```python
from build123d import *

# Parameters (mm, degrees)
SKETCH1_W           = 39.1
SKETCH1_H           = 23
BOSS_EXTRUDE1_DEPTH = 5.5
CUT_EXTRUDE1_DEPTH  = 26.208183195
FILLET1_R           = 6.35
FILLET2_R           = 0.5
SKETCH3_W           = 9
SKETCH3_H           = 9
BOSS_EXTRUDE2_DEPTH = 6.35


with BuildPart() as part:
    # Sketch1 → Boss-Extrude1 (new, symmetric)
    with BuildSketch(Plane.XY):
        Rectangle(SKETCH1_W, SKETCH1_H)
    extrude(amount=BOSS_EXTRUDE1_DEPTH, both=True)

    # Sketch2 → Cut-Extrude1 (cut, through all)
    with BuildSketch(Plane.XY.offset(5.5)):
        Polygon((19.55, -11.5), (-2.05, -11.5), (-2.05, -0.389755132), (19.55, 1.5), align=None)
    extrude(amount=-CUT_EXTRUDE1_DEPTH, mode=Mode.SUBTRACT)

    # Fillet1
    fillet1_edges = [part.edges().sort_by_distance(p)[0] for p in [
        (-2.05, -0.389755132, 0),
    ]]
    fillet(fillet1_edges, radius=FILLET1_R)

    # Fillet2
    fillet2_edges = [part.edges().sort_by_distance(p)[0] for p in [
        (0, 11.5, 5.5),
        (19.55, 6.5, -5.5),
        (19.55, 6.5, 5.5),
        (19.55, 1.5, 0),
        (-2.05, -11.5, 0),
        (11.648280517, 0.808689123, -5.5),
        (11.648280517, 0.808689123, 5.5),
        (-2.05, -8.854229044, 5.5),
        (-2.05, -8.854229044, -5.5),
        (-0.381711089, -1.918460269, 5.5),
        (-0.381711089, -1.918460269, -5.5),
        (-19.55, 0, 5.5),
        (0, 11.5, -5.5),
        (-10.8, -11.5, -5.5),
        (-19.55, 0, -5.5),
        (-10.8, -11.5, 5.5),
        (-19.55, 11.5, 0),
        (19.55, 11.5, 0),
        (-19.55, -11.5, 0),
    ]]
    fillet(fillet2_edges, radius=FILLET2_R)

    # Sketch3 → Boss-Extrude2 (add)
    with BuildSketch(Plane(origin=(19.55, 0, 0), x_dir=(0, 0, -1), z_dir=(1, 0, 0))):
        with Locations((0, 6.479082794)):
            Rectangle(SKETCH3_W, SKETCH3_H)
    extrude(amount=BOSS_EXTRUDE2_DEPTH)


solid = part.part
```
Build history of the part. All positions in model axes, mm. A direction names the side the tool comes from. Coordinates: 2 decimals unless noted, no trailing zeros. Order: outer loops, then holes, each group sorted by start corner. A loop starts at its lowest first (then second) coordinate and runs counter-clockwise, first axis right, second up. Notation, with made-up numbers: M 56,-16 L 74,-16 A20 ccw 74,-4 Z; hole C -4,51 d6. An arc over 180 degrees is marked long. One line per question, with ' | ' between items. Start each with the question number.
1. Wall check: line 1 along Y through (x, z) = (9.5, 0); line 2 along X through (y, z) = (-9.25, 0.75); line 3 along Y through (x, z) = (20, -3.75). Give the ranges that are in metal, low to high. Write a range as [from, to].
2. Flat gauge pins, fed straight in: P1, Ø3, axis at x = 22, z = 0, coming from the -Y side; P2, Ø1.9, axis at x = 23.5, z = -1, coming from the +Y side; P3, Ø4, axis at y = -9, z = -2.5, coming from the +X side. Where does each tip first touch, or does it go through?
3. Cut at B-B (y = 4). Write the cut outline in (x, z).
4. Tool access for faces 1 (the face through (23, 1.979, 0)), 2 (the face through (23, 6, -4.5)), 3 (the face through (23, 6, 4.5)), 4 (the face through (23, 10.979, 0)): list every direction of +Z, -Z, +X, -X, +Y, -Y with a clear straight run to the whole face (end or side of a thin tool).
The answers:
1) line 1: y = [0.62, 11.5] | line 2: x = [-19.55, -2.05] | line 3: y = [1.98, 10.98]
2) P1: stops at y = 1.98 | P2: stops at y = 10.98 | P3: stops at x = -2.05
3) outline: M -19.55,-5 A0.5 ccw -19.05,-5.5 L 19.05,-5.5 A0.5 ccw 19.55,-5 L 19.55,-4.5 L 25.9,-4.5 L 25.9,4.5 L 19.55,4.5 L 19.55,5 A0.5 ccw 19.05,5.5 L -19.05,5.5 A0.5 ccw -19.55,5 Z
4) face 1: +Z, -Z, +X, -Y | face 2: -Z, +X, +Y, -Y | face 3: +Z, +X, +Y, -Y | face 4: +Z, -Z, +X, +Y
